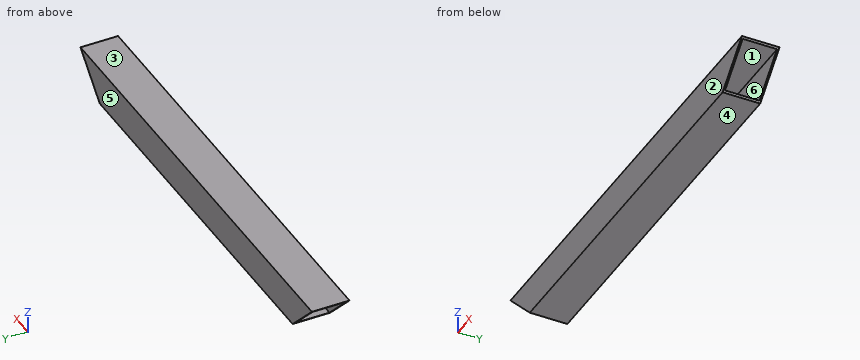
```python
from build123d import *

# Parameters (mm, degrees)
F0_W          = 76.2
F0_H          = 76.2
F0_W_2        = 69.85
F0_H_2        = 69.85
F1_DEPTH      = 457.2
F1_DEPTH_BACK = 457.2
F3_DEPTH      = 76.201


with BuildPart() as f1:
    # F0 (on Right) → F1 (new body, two sides)
    with BuildSketch(Plane.YZ) as f1_sk:
        Rectangle(F0_W, F0_H)
        Rectangle(F0_W_2, F0_H_2, mode=Mode.SUBTRACT)
    extrude(amount=F1_DEPTH)
    extrude(f1_sk.sketch, amount=-F1_DEPTH_BACK)

    # F2 (on face) → F3 (cut, through all)
    with BuildSketch(Plane.XZ.offset(38.1)):
        Polygon((-381, -38.1), (-457.2, 38.1), (-457.2, -38.1), align=None)
        Polygon((457.2, -38.1), (457.2, 38.1), (381, -38.1), align=None)
    extrude(amount=-F3_DEPTH, mode=Mode.SUBTRACT)


solid = f1.part
```
CAD build for the part. Positions are in the model's coordinates, mm. Face numbers are marked on the shaded views. A direction names the side the tool comes from. Round coordinates to 2 decimals unless told otherwise and drop trailing zeros. Write each loop counter-clockwise with the first axis right and the second up, starting at its lowest first coordinate (ties: lowest second). Pieces come first, ordered by that corner, then holes.
Item 1: Tool access for the marked faces 5 and 6: list every direction of +Z, -Z, +X, -X, +Y, -Y with a clear straight run to the whole face (end or side of a thin tool).
Filled in:
face 5: +Z, -Z, +X, -X, +Y
face 6: +X, -X
Item 2: Drill centre lines: L1, parallel to Y at x = 375.5, z = -14.5 (3 decimals); L2, parallel to Z at x = -393, y = 27 (3 decimals). Where is each one in solid material? Low to high.
Filled in:
L1: y = -38.1 to -34.925, 34.925 to 38.1
L2: z = 34.925 to 38.1
Item 3: Band-saw the part on C-C on y = 7. Write the cut outline in (x, z) (3 decimals).
Filled in:
outline: (-457.2, 38.1) - (-454.025, 34.925) - (454.025, 34.925) - (457.2, 38.1) - close; (-384.175, -34.925) - (-381, -38.1) - (381, -38.1) - (384.175, -34.925) - close
Item 4: Band-saw the part on B-B on x = -167. Write the cut outline in (y, z) (3 decimals), then the cut area to 3 significant figures.
Filled in:
outline: (-38.1, -38.1) - (38.1, -38.1) - (38.1, 38.1) - (-38.1, 38.1) - close; hole (-34.925, -34.925) - (34.925, -34.925) - (34.925, 34.925) - (-34.925, 34.925) - close
area: 927 mm2
Item 5: Band-saw the part on D-D on x = -396. Write the cut outline in (y, z) (3 decimals), then the cut area to 3 significant figures.
Filled in:
outline: (-38.1, -23.1) - (-34.925, -23.1) - (-34.925, 34.925) - (34.925, 34.925) - (34.925, -23.1) - (38.1, -23.1) - (38.1, 38.1) - (-38.1, 38.1) - close
area: 610 mm2
Item 6: Band-saw the part on A-A on z = 18. Write the cut outline in (x, y) (3 decimals).
Filled in:
outline: (-437.1, -38.1) - (437.1, -38.1) - (437.1, -34.925) - (-437.1, -34.925) - close; (-437.1, 34.925) - (437.1, 34.925) - (437.1, 38.1) - (-437.1, 38.1) - close
Item 7: Mould opens along Z. For the marked faces 1, 2, 3 and 4 say: released by +Z, released by -Z, zero draft, split by the parting line, or undercut.
Filled in:
face 1: undercut
face 2: zero draft
face 3: released by +Z
face 4: released by -Z
